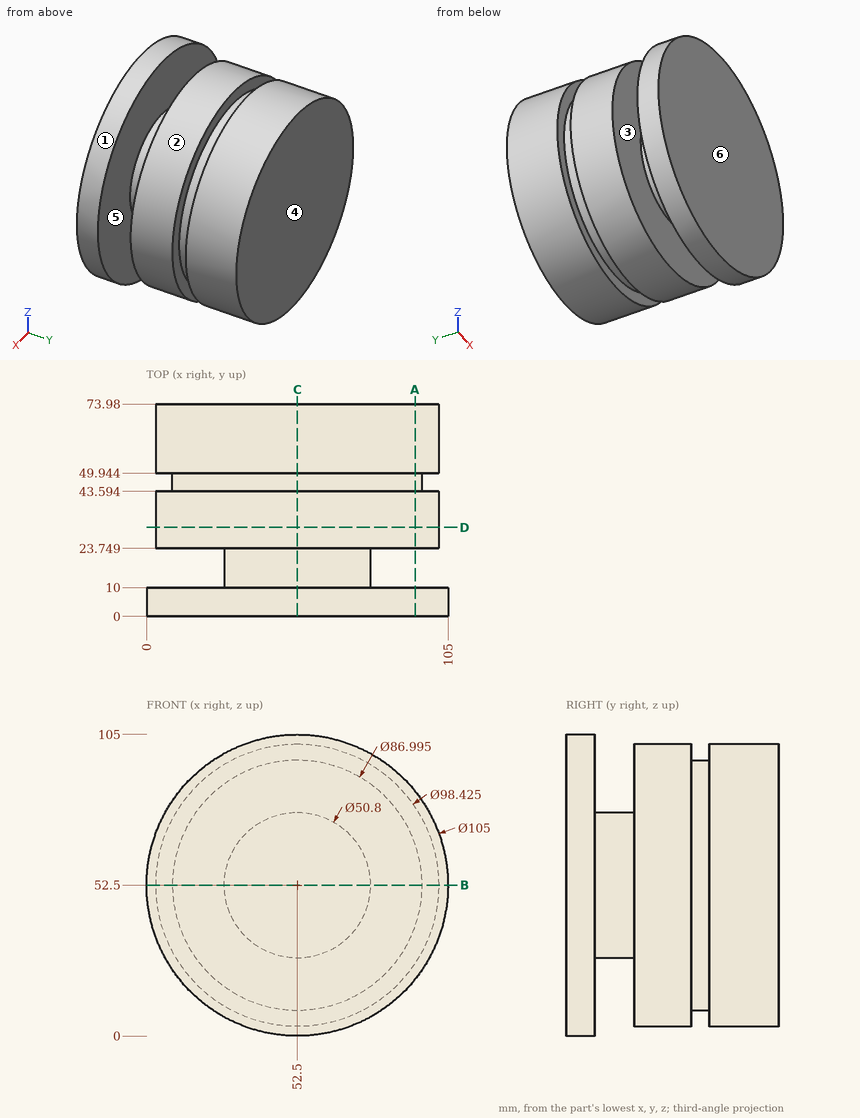
Geometry: see drawing. Coordinates: mm, zero at the bounding-box minimum. A direction names the side the tool comes from. Coordinates: 2 decimals unless noted, no trailing zeros. Order: outer loops, then holes, each group sorted by start corner. A loop starts at its lowest first (then second) coordinate and runs counter-clockwise, first axis right, second up. Notation, with made-up numbers: (86.25, 14) -> (130.25, 14) arc R12 cw to (130.25, 23) -> close; hole circle Ø8 at (-4.5, 0). An arc over 180 degrees is marked (long way). Write each question's results on one line, items separated by ' | '. Start each with the question number.
1) First-contact query: pin 1 (5 mm diameter, centred on y = 14, z = 49.5, fed in from -X) (3 decimals); pin 2 (6 mm diameter, centred on x = 84, y = 36.5, fed in from -Z); pin 3 (4 mm diameter, centred on y = 23.5, z = 53.5, fed in from -X). Flat tips, straight axial feed; report the tip coordinate or a pass-through.
2) Set-up query: the marked faces 1 and 2. Return all of +Z, -Z, +X, -X, +Y, -Y with unobstructed straight access to the full face (end or side cutting, diameter ignored); none if empty.
3) Cut plane A-A, the plane x = 93.5. Output: boundary loops of the cut face in (y, z).
4) Cut plane C-C, the plane x = 52.5. Output: boundary loops of the cut face in (y, z), and give its area (3 significant figures).
5) Mould query, pull axis Y, two halves, no side actions, for the marked faces 3, 4, 5 and 6. Classes: released by +Y, released by -Y, zero draft, split by the parting line, or undercut.
6) Cut plane B-B, the plane z = 52.5. Output: boundary loops of the cut face in (x, y).
7) Material intervals for line 1 along Y through (x, z) = (44, 6); line 2 along Y through (x, z) = (21.5, 27.5); line 3 along X through (y, z) = (63, 23.5), sorted ascending.
8) Cut plane D-D, the plane y = 31. Output: boundary loops of the cut face in (x, z) (1 decimal), and give its area (3 significant figures).
Checks:
1) pin 1: x = 27.105 | pin 2: z = 12.38 | pin 3: x = 3.29
2) face 1: +Y, -Y | face 2: +Y
3) outline: (0, 19.71) -> (10, 19.71) -> (10, 85.29) -> (0, 85.29) -> close; (23.75, 25.28) -> (43.59, 25.28) -> (43.59, 37.97) -> (49.94, 37.97) -> (49.94, 25.28) -> (73.98, 25.28) -> (73.98, 79.72) -> (49.94, 79.72) -> (49.94, 67.03) -> (43.59, 67.03) -> (43.59, 79.72) -> (23.75, 79.72) -> close
4) outline: (0, 0) -> (10, 0) -> (10, 27.1) -> (23.75, 27.1) -> (23.75, 3.29) -> (43.59, 3.29) -> (43.59, 9) -> (49.94, 9) -> (49.94, 3.29) -> (73.98, 3.29) -> (73.98, 101.71) -> (49.94, 101.71) -> (49.94, 96) -> (43.59, 96) -> (43.59, 101.71) -> (23.75, 101.71) -> (23.75, 77.9) -> (10, 77.9) -> (10, 105) -> (0, 105) -> close | area: 6,620 mm^2
5) face 3: undercut | face 4: released by +Y | face 5: undercut | face 6: released by -Y
6) outline: (0, 0) -> (105, 0) -> (105, 10) -> (77.9, 10) -> (77.9, 23.75) -> (101.71, 23.75) -> (101.71, 43.59) -> (96, 43.59) -> (96, 49.94) -> (101.71, 49.94) -> (101.71, 73.98) -> (3.29, 73.98) -> (3.29, 49.94) -> (9, 49.94) -> (9, 43.59) -> (3.29, 43.59) -> (3.29, 23.75) -> (27.1, 23.75) -> (27.1, 10) -> (0, 10) -> close
7) line 1: 0 to 10, 23.75 to 43.59, 49.94 to 73.98 | line 2: 0 to 10, 23.75 to 73.98 | line 3: 12.74 to 92.26
8) outline: circle Ø98.4 at (52.5, 52.5) | area: 7,610 mm^2
